Part model, mm, in its own coordinate system. A direction names the side the tool comes from. Give positions to 0.01 mm unless a question says otherwise; leave off trailing zeros. Order: outer loops, then holes, each group sorted by start corner. A loop starts at its lowest first (then second) coordinate and runs counter-clockwise, first axis right, second up. Notation, with made-up numbers: M -26,72.5 L -8,72.5 A24 cw -8,102.5 Z; hole C 35.25,45.25 d11. An arc over 180 degrees is marked long. Answer as a JSON object with one key per item and string values.
from build123d import *

# Parameters (mm, degrees)
F0_W     = 350
F0_H     = 30
F0_R     = 2.418964
F1_DEPTH = 2
F2_W     = 38.596436
F2_H     = 13.385396
F3_DEPTH = 15
F4_R     = 4.582497
F5_DEPTH = 21.693698


with BuildPart() as f1:
    # F0 (on Right) → F1 (new body)
    with BuildSketch(Plane.YZ):
        Rectangle(F0_W, F0_H)
        with Locations((-169.157952, 8.580949)):
            Circle(F0_R, mode=Mode.SUBTRACT)
    extrude(amount=F1_DEPTH)

    # F2 (on face) → F3 (join)
    with BuildSketch(Plane.YZ.offset(2)):
        Rectangle(F2_W, F2_H)
    extrude(amount=F3_DEPTH)

    # F4 (on face) → F5 (cut, through all)
    with BuildSketch(Plane.XY.offset(6.692698)):
        with Locations((9.614242, 0)):
            Circle(F4_R)
    extrude(amount=-F5_DEPTH, mode=Mode.SUBTRACT)


solid = f1.part
1. Cut at A-A on y = 0. Give the cut face in (x, z), plus the area to 3 significant figures.
Worked answers:
{"outline": "M 0,-15 L 2,-15 L 2,-6.69 L 5.03,-6.69 L 5.03,6.69 L 2,6.69 L 2,15 L 0,15 Z; M 14.2,-6.69 L 17,-6.69 L 17,6.69 L 14.2,6.69 Z", "area": "138 mm^2"}
2. Which spindle directions (+Z, -Z, +X, -X, +Y, -Y) get a long thin tool onto all of the face, cutting with end or side? Do faces 4 (the flat face through (8, -5, 6.693)), 5 (the flat face through (9, 19.298, 0)), 6 (the flat face through (8, -5, -6.693)). Say none if no direction does.
Worked answers:
{"face 4": "+Z, +X, +Y, -Y", "face 5": "+Z, -Z, +X, +Y", "face 6": "-Z, +X, +Y, -Y"}
3. Cut at D-D on y = 70. Give the cut face in (x, z), plus the area to 3 significant figures.
Worked answers:
{"outline": "M 0,-15 L 2,-15 L 2,15 L 0,15 Z", "area": "60.0 mm^2"}
4. Cut at C-C on z = -10. Give the cut face in (x, y), plus the area to 3 significant figures.
Worked answers:
{"outline": "M 0,-175 L 2,-175 L 2,175 L 0,175 Z", "area": "700 mm^2"}
5. Cut at B-B on x = 9.5. Give the cut face in (y, z).
Worked answers:
{"outline": "M -19.3,-6.69 L -4.58,-6.69 L -4.58,6.69 L -19.3,6.69 Z; M 4.58,-6.69 L 19.3,-6.69 L 19.3,6.69 L 4.58,6.69 Z"}
6. Two-plate mould, pull along Y, no slides. Class faces 1 (the flat face through (9, -19.298, 0)), 2 (the flat face through (0, -2, 0)), 3 (the cylindrical face through (5.036, 0.201, 0.094)): +Y half, -Y half, draft (parallel to the pull), parting line (faces both ways), or undercut.
Worked answers:
{"face 1": "-Y half", "face 2": "draft", "face 3": "undercut"}
7. Probe line 1 along Y through (x, z) = (3, 2); line 2 along X through (y, z) = (85.5, -3.25); line 3 along Z through (x, y) = (12, -8.5). List the from-to ranges inside material, lowest first.
Worked answers:
{"line 1": "y = -19.3 to 19.3", "line 2": "x = 0 to 2", "line 3": "z = -6.69 to 6.69"}
8. Pin check, flat tips, straight feed: P1, Ø5, axis at x = 11, z = -4, coming from the -Y side; P2, Ø1.5, axis at x = 11, y = -7, coming from the +Z side; P3, Ø5, axis at y = -42, z = 1, coming from the +X side. Stop position of each tip, or through.
Worked answers:
{"P1": "stops at y = -19.3", "P2": "stops at z = 6.69", "P3": "stops at x = 2"}
